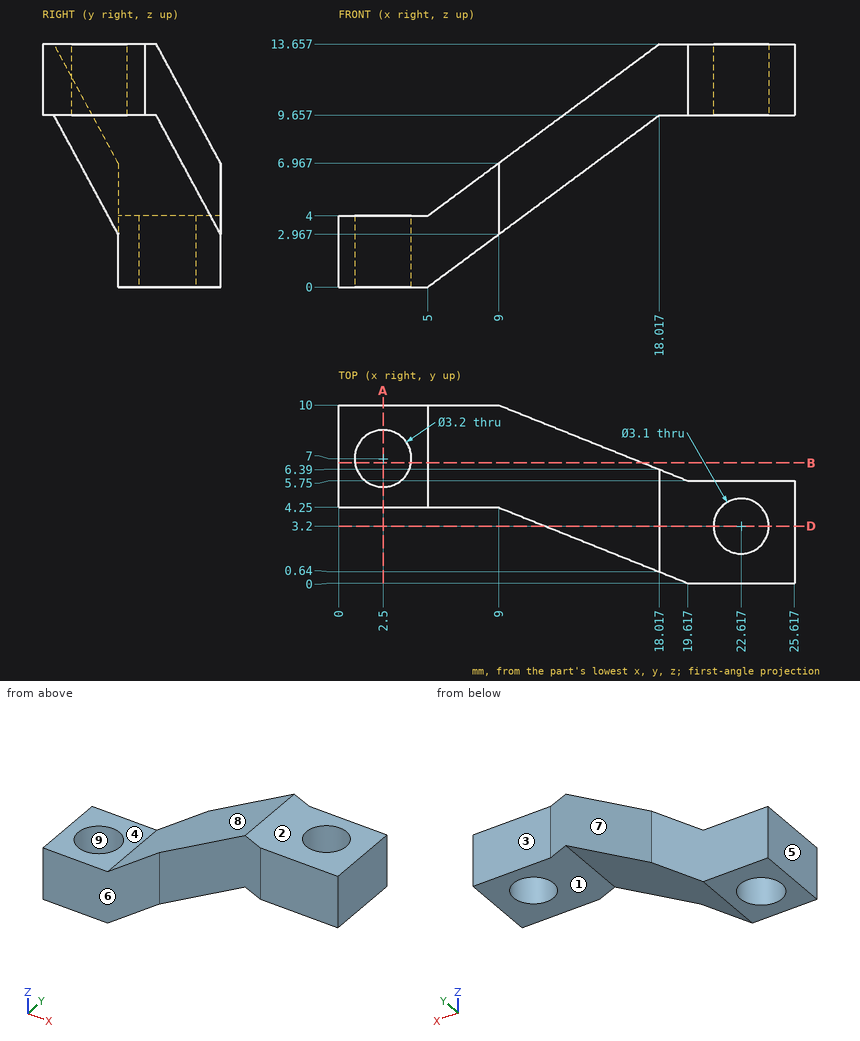
The drawing under review shows one solid part. Ordinate dimensions are in mm from its lowest x, y, z. A direction names the side the tool comes from. Round coordinates to 2 decimals unless told otherwise and drop trailing zeros. Loops run counter-clockwise (first coordinate to the right, second up) from the corner with the lowest first, then second, coordinate; pieces in that order, holes last. Notation, with made-up numbers: (-35.75, 66.5) - (-7.75, 66.5) arc R3 ccw to (-7.75, 70.5) - close; hole circle Ø6 at (-35.75, 29.25). An arc over 180 degrees is marked (long way). Use one line per item in the form item = value.
Item 1: Mouldability with a two-part tool opening along Y and no side actions: class the marked faces 6, 7, 8 and 9 as +Y half, -Y half, draft (parallel to the pull), parting line (faces both ways), or undercut.
Answers:
face_6 = -Y half
face_7 = +Y half
face_8 = draft
face_9 = undercut
Item 2: For line 1 (Y direction, x = 2.5, z = 2.3); line 2 (Z direction, x = 21, y = 5.5); line 3 (X direction, y = 2.25, z = 11.5) (1 decimal), list the stretches that pass through material, from the lowest coordinate up.
Answers:
line_1 = 4.25 to 5.4, 8.6 to 10
line_2 = 9.66 to 13.66
line_3 = 15.1 to 21.4, 23.8 to 25.6
Item 3: Consider section D-D on y = 3.2. Write out the cut boundary in (x, z).
Answers:
outline = (11.62, 4.91) - (18.02, 9.66) - (21.07, 9.66) - (21.07, 13.66) - (18.02, 13.66) - (11.62, 8.91) - close; (24.17, 9.66) - (25.62, 9.66) - (25.62, 13.66) - (24.17, 13.66) - close
Item 4: Consider section B-B on y = 6.75. Write out the cut boundary in (x, z).
Answers:
outline = (0, 0) - (0.92, 0) - (0.92, 4) - (0, 4) - close; (4.08, 0) - (5, 0) - (17.12, 8.99) - (17.12, 12.99) - (5, 4) - (4.08, 4) - close
Item 5: Consider section A-A on x = 2.5. Write out the cut boundary in (y, z), then the cut area to 3 significant figures.
Answers:
outline = (4.25, 0) - (5.4, 0) - (5.4, 4) - (4.25, 4) - close; (8.6, 0) - (10, 0) - (10, 4) - (8.6, 4) - close
area = 10.2 mm^2
Item 6: Tool access review of the marked faces 1, 2, 3, 4 and 5: name each direction out of +Z, -Z, +X, -X, +Y, -Y from which nothing blocks a thin tool from reaching the whole face with its end or side.
Answers:
face_1 = -Z, +X, +Y, -Y
face_2 = +Z, +X, -X, +Y, -Y
face_3 = +Z, -Z, +X, +Y
face_4 = +Z, -X, +Y, -Y
face_5 = +Z, -Z, -X, +Y, -Y
Item 7: Clearance check with flat-ended pins moving along their axes: P1, Ø3, axis at x = 20.5, y = 2, coming from the -Z side; P2, Ø1, axis at x = 17, y = 3, coming from the -Z side; P3, Ø1, axis at y = 5.5, z = 11.5, coming from the -X side (1 decimal). State where each tip first meets the part, or that it passes through.
Answers:
P1 = 9.66
P2 = 8.53
P3 = 14.4
